from build123d import *

# Parameters (mm, degrees)
SKETCH1_R           = 12.7
BOSS_EXTRUDE1_DEPTH = 5.08
SKETCH2_W           = 3.556
SKETCH2_H           = 2.604656918
SKETCH2_H_2         = 2.54
BOSS_EXTRUDE2_DEPTH = 19.05


with BuildPart() as part:
    # Sketch1 → Boss-Extrude1 (new body)
    with BuildSketch(Plane(origin=(0, 0, 0), x_dir=(1, 0, 0), z_dir=(0, 1, 0))):
        Circle(SKETCH1_R)
    extrude(amount=BOSS_EXTRUDE1_DEPTH)

    # Sketch2 → Boss-Extrude2 (add)
    with BuildSketch(Plane(origin=(0, 5.08, 0), x_dir=(1, 0, 0), z_dir=(0, 1, 0))):
        with Locations((0, 3.842328459)):
            Rectangle(SKETCH2_W, SKETCH2_H)
        with Locations((0, -3.81)):
            Rectangle(SKETCH2_W, SKETCH2_H_2)
    extrude(amount=BOSS_EXTRUDE2_DEPTH)


solid = part.part
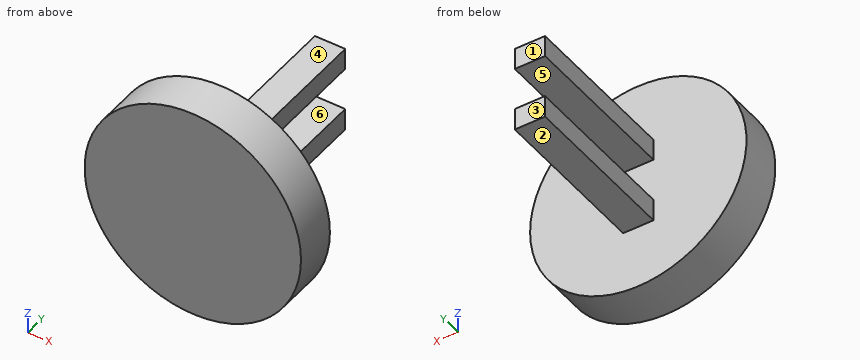
Design review of the part built by this model. Coordinates are the model's own, in mm. Face numbers are marked on the shaded views. A direction names the side the tool comes from. Coordinates: 2 decimals unless noted, no trailing zeros. Order: outer loops, then holes, each group sorted by start corner. A loop starts at its lowest first (then second) coordinate and runs counter-clockwise, first axis right, second up.
Item 1: For pin 1 Ø1 at (x, z) = (8, 3) entering from +Y; pin 2 Ø8 at (y, z) = (4.5, -6.5) entering from +X; pin 3 Ø6 at (y, z) = (4.5, 10) entering from -X; pin 4 Ø1.5 at (y, z) = (16.5, -6.5) entering from -X, all flat-tipped, find the tip position at first contact; note any pin that passes through.
Item 2: For the marked faces 1 and 2, list the 3-axis set-ups (+Z, -Z, +X, -X, +Y, -Y) from which the entire face can be reached by the end or side of a thin tool; tool diameter is ignored.
Item 3: The part is to be moulded in two halves that separate along Z. For the marked faces 3, 4, 5 and 6, say which applies: pulls with the +Z half, pulls with the -Z half, needs draft (parallel to the pull), parting line crosses it, or undercut.
Item 4: Take a section at D-D, the plane y = 3. Write out the cut boundary in (x, z).
Item 5: Take a section at A-A, the plane y = 13. Write out the cut boundary in (x, z), then the cut area to 3 significant figures.
Item 6: Take a section at B-B, the plane x = 0. Write out the cut boundary in (y, z).
Item 7: Take a section at C-C, the plane z = -4.75. Write out the cut boundary in (x, y), then the cut area to 3 significant figures.
Item 8: For line 1 (Z direction, x = -1.25, y = 15.75); line 2 (Y direction, x = 6, z = 1.5); line 3 (X direction, y = 7.75, z = 3), list the stretches that pass through material, from the lowest coordinate up.
The answers:
1. pin 1: stops at y = 5.08
1. pin 2: stops at x = 12.45
1. pin 3: stops at x = -10.6
1. pin 4: passes through
2. face 1: +Z, -Z, +X, -X, +Y
2. face 2: -Z, +X, -X, +Y
3. face 3: needs draft
3. face 4: pulls with the +Z half
3. face 5: undercut
3. face 6: undercut
4. outline: circle Ø25.4 at (0, 0)
5. outline: (-1.78, -5.14) - (1.78, -5.14) - (1.78, -2.54) - (-1.78, -2.54) - close; (-1.78, 2.54) - (1.78, 2.54) - (1.78, 5.08) - (-1.78, 5.08) - close
5. area: 18.3 mm2
6. outline: (0, -12.7) - (5.08, -12.7) - (5.08, -5.14) - (24.13, -5.14) - (24.13, -2.54) - (5.08, -2.54) - (5.08, 2.54) - (24.13, 2.54) - (24.13, 5.08) - (5.08, 5.08) - (5.08, 12.7) - (0, 12.7) - close
7. outline: (-11.78, 0) - (11.78, 0) - (11.78, 5.08) - (1.78, 5.08) - (1.78, 24.13) - (-1.78, 24.13) - (-1.78, 5.08) - (-11.78, 5.08) - close
7. area: 187 mm2
8. line 1: z = -5.14 to -2.54, 2.54 to 5.08
8. line 2: y = 0 to 5.08
8. line 3: x = -1.78 to 1.78
